Model file for the job. Use its own axes, mm. Coordinates: 2 decimals unless noted, no trailing zeros. Write each loop counter-clockwise with the first axis right and the second up, starting at its lowest first coordinate (ties: lowest second). Pieces come first, ordered by that corner, then holes. Notation, with made-up numbers: (5.5, 35) - (57.5, 35) arc R23 ccw to (57.5, 51) - close; hole circle Ø9 at (-6.5, -21). An arc over 180 degrees is marked (long way). Put each result on its own line as item: value. Start each with the question number.
1. Saw through at A-A, the plane x = 80. Write the cut outline in (y, z).
2. Drop a flat-ended pin along its axis: P1, Ø3, axis at x = 35, z = 5, coming from the +Y side. Give the stop position or say it passes through.
3. Saw through at B-B, the plane y = -4.9. Give the number of separate pieces and of enclosed holes in the cut face, plus the area to 3 significant figures.
4. Drill centre lines: L1, parallel to X at y = -5.55, z = -26; L2, parallel to Z at x = 0, y = -4.15; L3, parallel to X at y = -1.8, z = 25.5. Where is each one in solid material? Low to high. Write a range as from..to.
```python
from build123d import *

# Parameters (mm, degrees)
F0_W     = 180
F0_H     = 80
F0_R     = 3
F1_DEPTH = 6
F2_R     = 5


with BuildPart() as f1:
    # F0 (on Front) → F1 (new body)
    with BuildSketch(Plane.XZ):
        with Locations((0, 4.415482)):
            Rectangle(F0_W, F0_H)
        with Locations((-80, -25.584518)):
            Circle(F0_R, mode=Mode.SUBTRACT)
        with Locations((-56.777846, -16.584518)):
            Circle(F0_R, mode=Mode.SUBTRACT)
        with Locations((0, -16.584518)):
            Circle(F0_R, mode=Mode.SUBTRACT)
        with Locations((51.876541, -16.584518)):
            Circle(F0_R, mode=Mode.SUBTRACT)
        with Locations((80, -25.584518)):
            Circle(F0_R, mode=Mode.SUBTRACT)
        with Locations((-80, 34.415482)):
            Circle(F0_R, mode=Mode.SUBTRACT)
        with Locations((-56.777846, 25.415482)):
            Circle(F0_R, mode=Mode.SUBTRACT)
        with Locations((0, 25.415482)):
            Circle(F0_R, mode=Mode.SUBTRACT)
        with Locations((51.876541, 25.415482)):
            Circle(F0_R, mode=Mode.SUBTRACT)
        with Locations((80, 34.415482)):
            Circle(F0_R, mode=Mode.SUBTRACT)
    extrude(amount=F1_DEPTH)

    # F2
    f2_edges = [f1.edges().sort_by_distance(p)[0] for p in [
        (-90, -3, 44.415482),
        (-90, -3, -35.584518),
        (90, -3, 44.415482),
        (90, -3, -35.584518),
    ]]
    fillet(f2_edges, radius=F2_R)


solid = f1.part
```
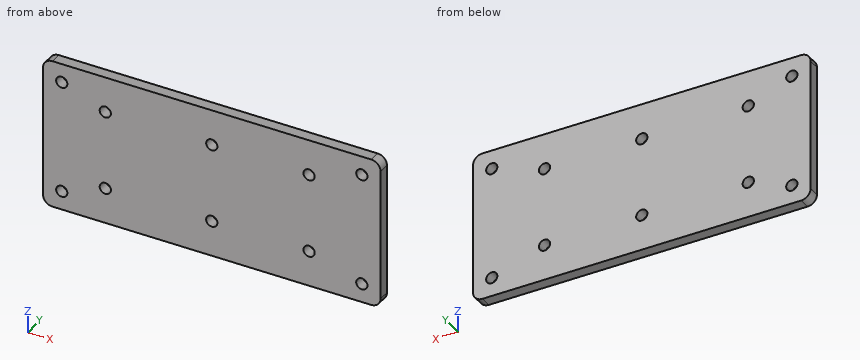
Final values:
1. outline: (-6, -35.58) - (0, -35.58) - (0, -28.58) - (-6, -28.58) - close; (-6, -22.58) - (0, -22.58) - (0, 31.42) - (-6, 31.42) - close; (-6, 37.42) - (0, 37.42) - (0, 44.42) - (-6, 44.42) - close
2. P1: stops at y = 0
3. separate pieces: 1
3. enclosed holes: 10
3. area: 14,100 mm²
4. L1: x = -90..-82.97, -77.03..77.03, 82.97..90
4. L2: z = -35.58..-19.58, -13.58..22.42, 28.42..44.42
4. L3: x = -90..-59.78, -53.78..-3, 3..48.88, 54.88..90
